from build123d import *

# Parameters (mm, degrees)
F0_W     = 254
F0_H     = 254
F0_R     = 38.1
F1_DEPTH = 76.2
F2_DEPTH = 203.2
F3_W     = 254
F3_H     = 254
F3_R     = 38.1
F4_DEPTH = 1270
F6_DEPTH = 1143
F7_R     = 50.8
F8_SIZE  = 25.4


with BuildPart() as f1:
    # F0 (on Top) → F1 (new body)
    with BuildSketch(Plane.XY):
        Rectangle(F0_W, F0_H)
        Circle(F0_R, mode=Mode.SUBTRACT)
        Circle(F0_R)
    extrude(amount=F1_DEPTH)

    # F0 (on Top) → F2 (join)
    with BuildSketch(Plane.XY):
        Circle(F0_R)
    extrude(amount=F2_DEPTH)

    # F3 (on face) → F4 (join)
    with BuildSketch(Plane.XY.offset(203.2)):
        Rectangle(F3_W, F3_H)
        Circle(F3_R)
    extrude(amount=F4_DEPTH)

    # F5 (on face) → F6 (cut)
    with BuildSketch(Plane.XY.offset(1473.2)):
        with BuildLine():
            Line((50.8, 0), (50.8, 50.8))
            Line((50.8, 50.8), (0, 50.8))
            ThreePointArc((0, 50.8), (35.921025, 35.921024), (50.8, 0))
        make_face()
        with BuildLine():
            Line((50.8, -50.8), (50.8, 0))
            ThreePointArc((50.8, 0), (35.921024, -35.921024), (0, -50.8))
            Line((0, -50.8), (50.8, -50.8))
        make_face()
        with BuildLine():
            ThreePointArc((0, -50.8), (-35.921024, -35.921025), (-50.8, 0))
            Line((-50.8, 0), (-50.8, -50.8))
            Line((-50.8, -50.8), (0, -50.8))
        make_face()
        with BuildLine():
            ThreePointArc((-50.8, 0), (-35.921025, 35.921024), (0, 50.8))
            Line((0, 50.8), (-50.8, 50.8))
            Line((-50.8, 50.8), (-50.8, 0))
        make_face()
        with BuildLine():
            ThreePointArc((50.8, 0), (35.921025, 35.921024), (0, 50.8))
            ThreePointArc((0, 50.8), (-35.921025, 35.921024), (-50.8, 0))
            ThreePointArc((-50.8, 0), (-35.921024, -35.921025), (0, -50.8))
            ThreePointArc((0, -50.8), (35.921024, -35.921024), (50.8, 0))
        make_face()
    extrude(amount=-F6_DEPTH, mode=Mode.SUBTRACT)

    # F7
    f7_edges = [f1.edges().sort_by_distance(p)[0] for p in [
        (-38.1, 0, 76.2),
        (-38.1, 0, 203.2),
    ]]
    fillet(f7_edges, radius=F7_R)

    # F8
    f8_edges = [f1.edges().sort_by_distance(p)[0] for p in [
        (0, -127, 76.2),
        (127, 0, 76.2),
        (0, 127, 76.2),
        (-127, 0, 76.2),
    ]]
    chamfer(f8_edges, length=F8_SIZE)


solid = f1.part
Design review of the part built by this model. Coordinates are the model's own, in mm. A direction names the side the tool comes from. Give positions to 0.01 mm unless a question says otherwise; leave off trailing zeros. Loops run counter-clockwise (first coordinate to the right, second up) from the corner with the lowest first, then second, coordinate; pieces in that order, holes last. Notation, with made-up numbers: M 11.5,-33.5 L 56.5,-33.5 A10 cw 56.5,-24.5 Z; hole C 57,-24.5 d3. An arc over 180 degrees is marked long. One line per question, with ' | ' between items. Start each with the question number.
1. Insertion check: P1, Ø6, axis at x = 2, z = 201.5, coming from the +Y side; P2, Ø2, axis at x = -10.5, y = -24, coming from the +Z side. Each pin has a flat end and moves straight along its axis. Give the tip position at first contact, or say it passes through.
2. For faces 1 (the face through (-50.8, 1, 910)), 2 (the face through (-1.8, 114.5, 63.3)), 3 (the face through (-86, 30, 203.2)), list the 3-axis set-ups (+Z, -Z, +X, -X, +Y, -Y) from which the entire face can be reached by the end or side of a thin tool; tool diameter is ignored.
3. Add section A-A (z = 847.5). Write out the cut boundary in (x, y).
4. The part is to be moulded in two halves that separate along Z. For faces 4 (the face through (1, 50.8, 910)), 5 (the face through (-1, 1, 330.2)), 6 (the face through (-114.5, -1.8, 63.3)), say which applies: released by +Z, released by -Z, zero draft, split by the parting line, or undercut.
5. Add section B-B (y = 0). Write out the cut boundary in (x, z), plus the area to 3 significant figures.
6. To check wall thickness, follow L1, parallel to Z at x = 62, y = 101; L2, parallel to X at y = 45, z = 857. State the ranges of each line that lie inside material, in increasing order.
Worked out:
1) P1: stops at y = 127 | P2: stops at z = 330.2
2) face 1: +Z | face 2: +X, -X, +Y | face 3: none
3) outline: M -127,-127 L 127,-127 L 127,127 L -127,127 Z; hole M -50.8,-50.8 L 50.8,-50.8 L 50.8,50.8 L -50.8,50.8 Z
4) face 4: zero draft | face 5: released by +Z | face 6: undercut
5) outline: M -127,0 L 127,0 L 127,50.8 L 101.6,76.2 L 88.9,76.2 A50.8 cw 38.1,127 L 38.1,152.4 A50.8 cw 88.9,203.2 L 127,203.2 L 127,1473.2 L 50.8,1473.2 L 50.8,330.2 L -50.8,330.2 L -50.8,1473.2 L -127,1473.2 L -127,203.2 L -88.9,203.2 A50.8 cw -38.1,152.4 L -38.1,127 A50.8 cw -88.9,76.2 L -101.6,76.2 L -127,50.8 Z | area: 237,000 mm²
6) L1: z = 0 to 76.2, 203.2 to 1473.2 | L2: x = -127 to -50.8, 50.8 to 127
